Can you work these out from the model? Positions are in its coordinate system, mm. A direction names the side the tool comes from. Give positions to 0.01 mm unless a question says otherwise; leave off trailing zeros. Order: outer loops, then holes, each group sorted by start corner. A loop starts at its lowest first (then second) coordinate and runs counter-clockwise, first axis right, second up. Notation, with made-up numbers: (53.25, 6) - (66.25, 6) arc R26 ccw to (66.25, 28) - close; hole circle Ø3 at (-30.75, -36). An arc over 180 degrees is marked (long way). Return JSON: item names as keys, results as strings.
```python
from build123d import *

# Parameters (mm, degrees)
BOSS_EXTRUDE1_DEPTH     = 111.76
SKETCH5_W               = 304.8
SKETCH5_H               = 25.4
CUT_EXTRUDE3_DEPTH      = 101.6
CUT_EXTRUDE4_DEPTH      = 227.288199427
CUT_EXTRUDE4_DEPTH_BACK = 227.288199427
SKETCH3_W               = 96.52
SKETCH3_H               = 101.6
SKETCH3_W_2             = 48.26


with BuildPart() as part:
    # Sketch1 → Boss-Extrude1 (new body)
    with BuildSketch(Plane.XY):
        Polygon((-152.4, 62.23), (-152.4, -33.02), (0, -62.23), (152.4, -32.976439839), (152.4, 62.23), align=None)
    extrude(amount=-BOSS_EXTRUDE1_DEPTH)

    # Sketch5 → Cut-Extrude3 (cut)
    with BuildSketch(Plane.XY.offset(-5.08)):
        with Locations((0, -1.27)):
            Rectangle(SKETCH5_W, SKETCH5_H)
    extrude(amount=-CUT_EXTRUDE3_DEPTH, mode=Mode.SUBTRACT)

    # Sketch3 → Cut-Extrude4 (cut, two sides: drawn at the far end of the back side and taken through both)
    with BuildSketch(Plane(origin=(0, 62.23, 0), x_dir=(1, 0, 0), z_dir=(0, 1, 0)).offset(-CUT_EXTRUDE4_DEPTH_BACK)):
        with Locations((-50.8, 55.88)):
            Rectangle(SKETCH3_W, SKETCH3_H)
        with Locations((50.8, 55.88)):
            Rectangle(SKETCH3_W, SKETCH3_H)
        with Locations((-128.27, 55.88)):
            Rectangle(SKETCH3_W_2, SKETCH3_H)
        with Locations((128.27, 55.88)):
            Rectangle(SKETCH3_W_2, SKETCH3_H)
    extrude(amount=CUT_EXTRUDE4_DEPTH + CUT_EXTRUDE4_DEPTH_BACK, mode=Mode.SUBTRACT)


solid = part.part
```
1. Thinking about a two-plate mould opening in X: for faces 1 (the face through (2.54, -38, -55)), 2 (the face through (1, 62.23, -56)), 3 (the face through (104.14, 36, -55)), 4 (the face through (-104.14, -28, -55)), which applies, +X half, -X half, draft (parallel to the pull), parting line (faces both ways), or undercut?
Checks:
{"face 1": "undercut", "face 2": "draft", "face 3": "+X half", "face 4": "-X half"}
2. If I drill on L1, parallel to X at y = -23, z = -32.5; L2, parallel to Z at x = 137, y = -2.5; L3, parallel to X at y = -43.5, z = -28, over which ranges is the centre line in solid material (lowest first)? Write a range as [from, to].
Checks:
{"L1": "[-104.14, -99.06], [-2.54, 2.54], [99.06, 104.14]", "L2": "[-111.76, -106.68], [-5.08, 0]", "L3": "[-2.54, 2.54]"}
3. Suppose I cut it at A-A (y = -5.5). List the corners of the cut face in (x, z) for me.
Checks:
{"outline": "(-152.4, -111.76) - (152.4, -111.76) - (152.4, -106.68) - (-152.4, -106.68) - close; (-152.4, -5.08) - (152.4, -5.08) - (152.4, 0) - (-152.4, 0) - close"}
4. On a 3-axis mill with a long thin cutter (end or side, diameter ignored), from which of +Z, -Z, +X, -X, +Y, -Y can I reach the whole of each face in a straight line? I mean faces 5 (the face through (99.06, 36, -55)), 6 (the face through (-2, 1, -111.76)), 7 (the face through (104.14, -28, -55)). Say none if no direction works.
Checks:
{"face 5": "+Y, -Y", "face 6": "-Z, +X, -X, +Y, -Y", "face 7": "+X, +Y, -Y"}
5. Suppose I cut it at D-D (x = -39). List the corners of the cut face in (y, z) for me (3 decimals).
Checks:
{"outline": "(-54.755, -111.76) - (62.23, -111.76) - (62.23, -106.68) - (-54.755, -106.68) - close; (-54.755, -5.08) - (62.23, -5.08) - (62.23, 0) - (-54.755, 0) - close"}
6. Suppose I cut it at B-B (z = -86.5). List the corners of the cut face in (x, y) for me, plus the area to 3 significant figures.
Checks:
{"outline": "(-104.14, -42.27) - (-99.06, -43.24) - (-99.06, -13.97) - (-104.14, -13.97) - close; (-104.14, 11.43) - (-99.06, 11.43) - (-99.06, 62.23) - (-104.14, 62.23) - close; (-2.54, -61.74) - (0, -62.23) - (2.54, -61.74) - (2.54, -13.97) - (-2.54, -13.97) - close; (-2.54, 11.43) - (2.54, 11.43) - (2.54, 62.23) - (-2.54, 62.23) - close; (99.06, -43.22) - (104.14, -42.24) - (104.14, -13.97) - (99.06, -13.97) - close; (99.06, 11.43) - (104.14, 11.43) - (104.14, 62.23) - (99.06, 62.23) - close", "area": "1,310 mm^2"}
7. Suppose I cut it at C-C (y = -18). List the corners of the cut face in (x, z) for me, plus the area to 3 significant figures.
Checks:
{"outline": "(-152.4, -111.76) - (152.4, -111.76) - (152.4, -106.68) - (104.14, -106.68) - (104.14, -5.08) - (152.4, -5.08) - (152.4, 0) - (-152.4, 0) - (-152.4, -5.08) - (-104.14, -5.08) - (-104.14, -106.68) - (-152.4, -106.68) - close; hole (-99.06, -106.68) - (-2.54, -106.68) - (-2.54, -5.08) - (-99.06, -5.08) - close; hole (2.54, -106.68) - (99.06, -106.68) - (99.06, -5.08) - (2.54, -5.08) - close", "area": "4,650 mm^2"}
8. For pin 1 Ø24 at (y, z) = (-41.5, -38.5) entering from +X; pin 2 Ø12 at (y, z) = (-39, -57) entering from -X; pin 3 Ø2.5 at (x, z) = (-101, -39.5) entering from -Y, each with a flat end and sliding along its axis, tell me the tip position at first contact or that it passes through.
Checks:
{"pin 1": "x = 104.14", "pin 2": "x = -104.14", "pin 3": "y = -43.11"}
